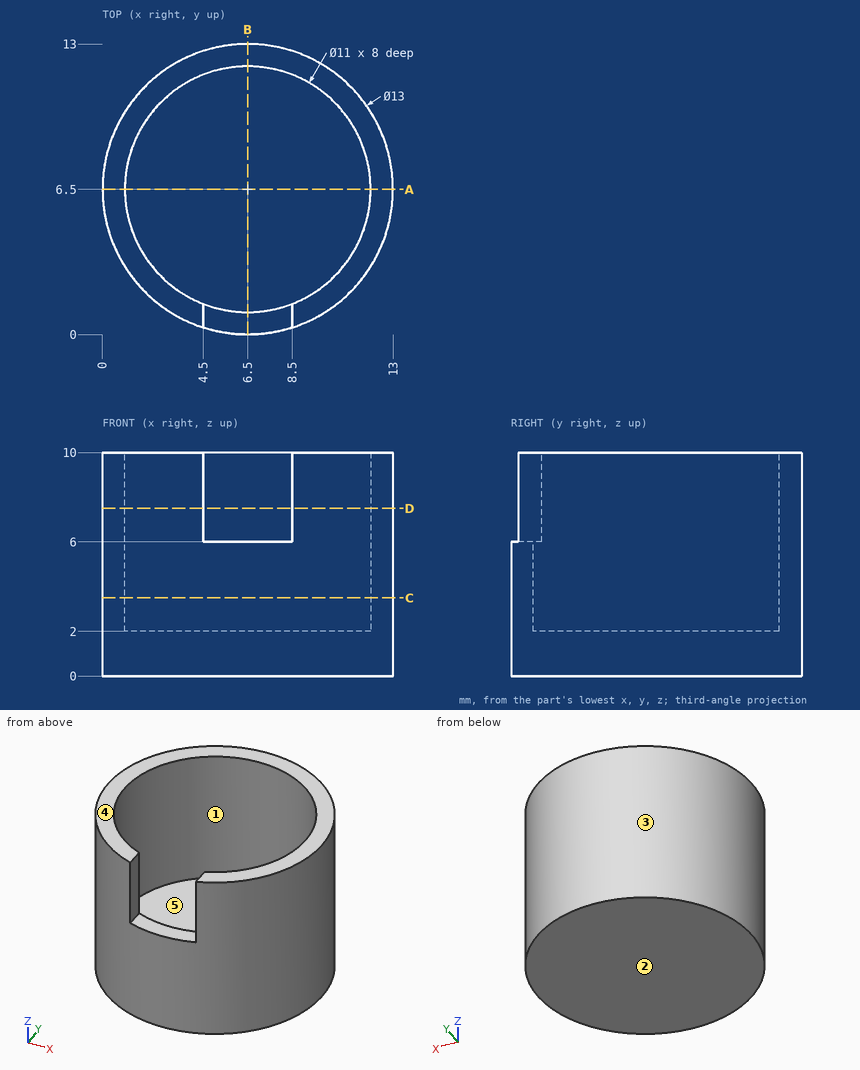
Job drawing, mm, ordinate dimensions from the low corner. One solid piece. A direction names the side the tool comes from. Give positions to 0.01 mm unless a question says otherwise; leave off trailing zeros. Write each loop counter-clockwise with the first axis right and the second up, starting at its lowest first coordinate (ties: lowest second). Pieces come first, ordered by that corner, then holes. Notation, with made-up numbers: M -29,80.5 L 19,80.5 A27 cw 19,99.5 Z; hole C 20.5,-31.75 d11. An arc over 180 degrees is marked long. One line per item, written item: value. Start each with the question number.
Q1. Saw through at D-D, the plane z = 7.5. Write the cut outline in (x, y), plus the area to 3 significant figures.
Q2. 3-axis set-ups, long thin cutter, end or side, ignore diameter. For the marked faces 4 and 5: which of +Z, -Z, +X, -X, +Y, -Y reach the whole face in a straight line?
Q3. Two-plate mould, pull along Y, no slides. Class the marked faces 1, 2 and 3: +Y half, -Y half, draft (parallel to the pull), parting line (faces both ways), or undercut.
Q4. Drop flat-ended pins along their axis: pin 1 Ø0.7 at (x, y) = (7, 0.5) entering from +Z; pin 2 Ø3 at (y, z) = (11.5, 2) entering from +X; pin 3 Ø0.8 at (y, z) = (1, 7.5) entering from -X. Give the stop position or say it passes through.
Q5. Saw through at B-B, the plane x = 6.5. Write the cut outline in (y, z).
Q6. Saw through at A-A, the plane y = 6.5. Write the cut outline in (x, z), plus the area to 3 significant figures.
Q7. Saw through at C-C, the plane z = 3.5. Write the cut outline in (x, y), plus the area to 3 significant figures.
Q8. Probe probe 1 along X at (y, z) = (6.5, 7.75); probe 2 along Z at (x, y) = (7.5, 6.25). List the from-to ranges inside material, lowest first. Write a range as [from, to].
Output values:
1. outline: M 4.5,0.32 L 4.5,1.38 A5.5 cw long 8.5,1.38 L 8.5,0.32 A6.5 ccw long Z
1. area: 33.6 mm²
2. face 4: +Z, +X, -X, +Y, -Y
2. face 5: +Z
3. face 1: undercut
3. face 2: draft
3. face 3: parting line
4. pin 1: stops at z = 6
4. pin 2: stops at x = 11.98
4. pin 3: stops at x = 2.47
5. outline: M 0,0 L 13,0 L 13,10 L 12,10 L 12,2 L 1,2 L 1,6 L 0,6 Z
6. outline: M 0,0 L 13,0 L 13,10 L 12,10 L 12,2 L 1,2 L 1,10 L 0,10 Z
6. area: 42.0 mm²
7. outline: C 6.5,6.5 d13; hole C 6.5,6.5 d11
7. area: 37.7 mm²
8. probe 1: x = [0, 1], [12, 13]
8. probe 2: z = [0, 2]
